Design review of the part built by this model. Coordinates are the model's own, in mm. A direction names the side the tool comes from. Give positions to 0.01 mm unless a question says otherwise; leave off trailing zeros. Order: outer loops, then holes, each group sorted by start corner. A loop starts at its lowest first (then second) coordinate and runs counter-clockwise, first axis right, second up.
Autodesk Inventor part; units mm, degrees
ref_plane "YZ Plane" through (0, 0, 0) normal (1, 0, 0) x (0, 1, 0)
ref_plane "XZ Plane" through (0, 0, 0) normal (0, 1, 0) x (-1, 0, 0)
ref_plane "XY Plane" through (0, 0, 0) normal (0, 0, 1) x (1, 0, 0)
sketch "スケッチ1" plane through (0, 0, 0) normal (0, 1, 0) x (-1, 0, 0)
  line L0 (0, -25) -> (42, -25)
  line L1 (42, -25) -> (42, 25)
  line L2 (42, 25) -> (0, 25)
  line L3 (0, 25) -> (0, -25)
  point P0 (0, 0)
  dimension "d0" = 42
  dimension "d1" = 50
  dimension "d40" = 25
extrude "プレート1" add sketch "スケッチ1" along normal blind 2
sketch "スケッチ4" plane through (0, 2, 0) normal (0, 1, 0) x (1, 0, 0)
  circle A0 centre (-25, 0) radius 11.1
  line L0 (0, 25) -> (0, -25)
  point P0 (0, 0)
  dimension "d23" = 22.2
  dimension "d24" = 25
extrude "押し出し1" cut sketch "スケッチ4" against normal blind 10
sketch "スケッチ5" plane through (0, 2, 0) normal (0, 1, 0) x (1, 0, 0)
  circle A0 centre (-25, 0) radius 11.1
  line L0 (0, 25) -> (0, -25)
  line L1 (-42, 25) -> (0, 25)
  line L2 (-42, -25) -> (-42, 25)
  line L3 (0, -25) -> (-42, -25)
  circle A1 centre (-25, 0) radius 14
  point P0 (0, 0)
  point P1 (-34.8995, -9.8995)
  point P2 (-15.1005, -9.8995)
  point P3 (-15.1005, 9.8995)
  point P4 (-34.8995, 9.8995)
  dimension "d28" = 28
  dimension "d31" = 360
hole "穴2" at (-34.8995, 2, 9.8995) at (-15.1005, 2, 9.8995) at (-15.1005, 2, -9.8995) at (-34.8995, 2, -9.8995) direction (0, -1, 0) diameter 3.2 end through all
sketch "スケッチ10" plane through (-2, 0, -25) normal (1, 0, 0) x (0, 1, 0)
  line L0 (0, 50) -> (0, 0)
  line L1 (0, 0) -> (20, 0)
  line L2 (20, 0) -> (20, 50)
  line L3 (20, 50) -> (0, 50)
edge flange "フランジ4" height 20 angle 90 thickness 2 bend radius 2 thickness toward (1, 0, 0) relief tear relief width 2 relief depth 1 edges at (0, 2, 0) wall of the first edge with corners at (-2, 0, 25) (-2, 0, -25) (-2, 20, -25) (-2, 20, 25)
bend "曲げ4"
corner "コーナー4"
sketch "スケッチ12" plane through (-2, 20, -25) normal (-1, 0, 0) x (0, 0, 1)
  line L0 (0, -16) -> (50, -16)
  line L1 (50, -16) -> (50, 0)
  line L2 (50, 0) -> (0, 0)
  line L3 (0, -16) -> (0, 0)
  line L4 (45, -10) -> (5, -10)
  point P0 (25, -20)
  point P1 (25, -10)
  dimension "d77" = 40
  dimension "d78" = 10
  dimension "d79" = 25
  dimension "d80" = 50
hole "穴3" at (-2, 10, -20) at (-2, 10, 20) direction (1, 0, 0) diameter 4.2 end through all
chamfer "面取り1" distance 10 angle 45 2 edges at (-42, 1, 25) (-42, 1, -25)
fillet "フィレット1" radius 2 4 edges at (-32, 1, -25) (-42, 1, -15) (-42, 1, 15) (-32, 1, 25)
chamfer "面取り2" distance 5 angle 45 2 edges at (-1, 20, -25) (-1, 20, 25)
fillet "フィレット2" radius 2 4 edges at (-1, 15, -25) (-1, 20, -20) (-1, 20, 20) (-1, 15, 25)
equation "\"d38\" = Thickness"
equation "\"d86\" = Thickness"
equation "\"d2\" = Thickness"
equation "\"d67\" = BendReliefWidth"
equation "\"d68\" = BendReliefDepth"
equation "\"d69\" = MinimumRemnant"
equation "\"d70\" = TransitionRadius"
equation "\"d73\" = BendRadius"
equation "\"d74\" = CornerReliefSize"
equation "\"d75\" = GapSize"
equation "\"d76\" = JacobiRadiusSize"
equation "\"BendRadius\" = Thickness"
equation "\"BendReliefWidth\" = Thickness"
equation "\"BendReliefDepth\" = 0.5 * Thickness"
equation "\"CornerReliefSize\" = 4 * Thickness"
equation "\"MinimumRemnant\" = 2 * Thickness"
equation "\"TransitionRadius\" = BendRadius"
equation "\"JacobiRadiusSize\" = BendRadius"
equation "\"GapSize\" = Thickness"
properties part number "Belt_Unit_Motor_Holder"
1. Take a section at D-D (z = 13). State the section outline as (x, y) points.
Recorded:
outline: (-42, 0) - (-4, 0) arc R4 ccw to (0, 4) - (0, 20) - (-2, 20) - (-2, 4) arc R2 cw to (-4, 2) - (-42, 2) - close
2. For pin 1 (6 mm diameter, centred on x = -17.5, z = -18, fed in from +Y); pin 2 (3 mm diameter, centred on y = 11.5, z = 3.5, fed in from -X), all flat-tipped, find the tip position at first contact; note any pin that passes through.
Recorded:
pin 1: stops at y = 2
pin 2: stops at x = -2
3. Draft analysis for pull direction Y (two halves, no side actions). For faces 3 (the face through (-0.986, 9.369, -17.997)), 4 (the face through (-0.986, 14.947, 24.844)), 5 (the face through (-37, 1, 20)), state which applies: pulls with the +Y half, pulls with the -Y half, needs draft (parallel to the pull), parting line crosses it, or undercut.
Recorded:
face 3: undercut
face 4: pulls with the +Y half
face 5: needs draft
4. Take a section at C-C (z = 0). State the section outline as (x, y) points, then the cut area to 3 significant figures.
Recorded:
outline: (-42, 0) - (-36.1, 0) - (-36.1, 2) - (-42, 2) - close; (-13.9, 0) - (-4, 0) arc R4 ccw to (0, 4) - (0, 20) - (-2, 20) - (-2, 4) arc R2 cw to (-4, 2) - (-13.9, 2) - close
area: 73.0 mm2
5. Take a section at A-A (x = -25). State the section outline as (y, z) points.
Recorded:
outline: (0, -25) - (2, -25) - (2, -11.1) - (0, -11.1) - close; (0, 11.1) - (2, 11.1) - (2, 25) - (0, 25) - close
6. Machinability: for faces 1 (the face through (-2, 12, 0)), 2 (the face through (0, 12, 0)), which of the approach directions +Z, -Z, +X, -X, +Y, -Y give a long, thin tool a straight path to every point of the face, cutting with its end or side? Answer none if there is none.
Recorded:
face 1: +Z, -Z, -X, +Y
face 2: +Z, -Z, +X, +Y, -Y
7. Take a section at B-B (y = 10). State the section outline as (x, z) points.
Recorded:
outline: (-2, -25) - (0, -25) - (0, -22.1) - (-2, -22.1) - close; (-2, -17.9) - (0, -17.9) - (0, 17.9) - (-2, 17.9) - close; (-2, 22.1) - (0, 22.1) - (0, 25) - (-2, 25) - close
8. For line 1 along Z through (x, y) = (-0.65, 10); line 2 along X through (y, z) = (17.5, 17); line 3 along Y through (x, z) = (-11.5, 11), list the stretches that pass through material, from the lowest coordinate up.
Recorded:
line 1: z = -25 to -22.1, -17.9 to 17.9, 22.1 to 25
line 2: x = -2 to 0
line 3: y = 0 to 2
